The drawing under review shows one solid part. Ordinate dimensions are in mm from its lowest x, y, z. A direction names the side the tool comes from. Give positions to 0.01 mm unless a question says otherwise; leave off trailing zeros. Write each loop counter-clockwise with the first axis right and the second up, starting at its lowest first coordinate (ties: lowest second). Pieces come first, ordered by that corner, then holes. Notation, with made-up numbers: (27, 49.25) -> (48, 49.25) arc R23 ccw to (48, 58.25) -> close; hole circle Ø4 at (66.5, 47). An arc over 180 degrees is marked (long way). Use CSV: the item, a comma, the result in double quotes.
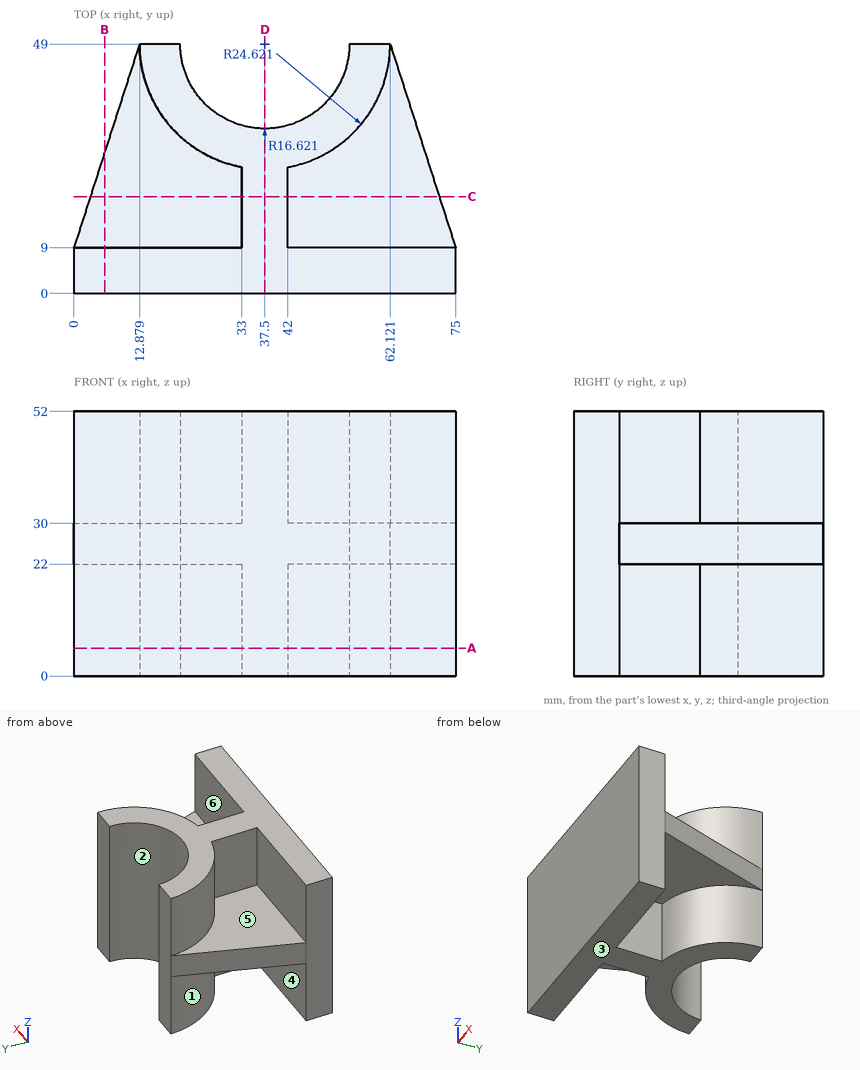
(1) For line 1 along Y through (x, z) = (64, 45.5); line 2 along X through (y, z) = (17, 9.5); line 3 along X through (y, z) = (39, 28.5), list the stretches that pass through material, from the lowest coordinate up. Write a range as [from, to].
Established:
line 1,"y = [0, 9]"
line 2,"x = [33, 42]"
line 3,"x = [9.66, 24.22], [50.78, 65.34]"
(2) Take a section at A-A (z = 5.5). Write out the cut boundary in (x, y).
Established:
outline,"(0, 0) -> (75, 0) -> (75, 9) -> (42, 9) -> (42, 24.79) arc R24.62 ccw to (62.12, 49) -> (54.12, 49) arc R16.62 cw to (20.88, 49) -> (12.88, 49) arc R24.62 ccw to (33, 24.79) -> (33, 9) -> (0, 9) -> close"
(3) Tool access review of the marked faces 4, 5 and 6: name each direction out of +Z, -Z, +X, -X, +Y, -Y from which nothing blocks a thin tool from reaching the whole face with its end or side.
Established:
face 4,"-Z, -X"
face 5,"+Z, -X"
face 6,"+Z, +X"
(4) Clearance check with flat-ended pins moving along their axes: pin 1 (3 mm diameter, centred on y = 25, z = 34.5, fed in from -X); pin 2 (5 mm diameter, centred on y = 34.5, z = 24, fed in from -X) (1 decimal); pin 3 (16.5 mm diameter, centred on x = 19.5, y = 32, fed in from +Z); pin 4 (5 mm diameter, centred on x = 62, y = 31, fed in from -Z). State where each tip first meets the part, or that it passes through.
Established:
pin 1,"stops at x = 27.5"
pin 2,"stops at x = 7.4"
pin 3,"stops at z = 52"
pin 4,"stops at z = 22"
(5) Take a section at B-B (x = 6). Write out the cut boundary in (y, z) (1 decimal), then the cut area to 3 significant figures.
Established:
outline,"(0, 0) -> (9, 0) -> (9, 22) -> (27.6, 22) -> (27.6, 30) -> (9, 30) -> (9, 52) -> (0, 52) -> close"
area,"617 mm2"
(6) Mouldability with a two-part tool opening along Y and no side actions: class the marked faces 1, 2 and 3 as +Y half, -Y half, draft (parallel to the pull), parting line (faces both ways), or undercut.
Established:
face 1,"undercut"
face 2,"+Y half"
face 3,"draft"
(7) Take a section at C-C (y = 19). Write out the cut boundary in (x, z).
Established:
outline,"(3.22, 22) -> (33, 22) -> (33, 0) -> (42, 0) -> (42, 22) -> (71.78, 22) -> (71.78, 30) -> (42, 30) -> (42, 52) -> (33, 52) -> (33, 30) -> (3.22, 30) -> close"
(8) Take a section at D-D (x = 37.5). Write out the cut boundary in (y, z).
Established:
outline,"(0, 0) -> (32.38, 0) -> (32.38, 52) -> (0, 52) -> close"
